The listing builds one solid part. Answer for the finished solid, in the listing's coordinates (mm). Face numbers are marked on the shaded views. Give positions to 0.01 mm unless a question says otherwise; leave off trailing zeros. Order: outer loops, then holes, each group sorted by start corner. A loop starts at its lowest first (then second) coordinate and runs counter-clockwise, first axis right, second up. Notation, with made-up numbers: (35.25, 56) - (65.25, 56) arc R28 cw to (65.25, 77) - close; hole circle Ø10 at (-20.5, 58.5). An arc over 180 degrees is marked (long way). Answer in a Markdown table with one row per item.
from build123d import *

# Parameters (mm, degrees)
BOSS_EXTRUDE2_DEPTH                                 = 5
CSK_FOR_M3_COUNTERSUNK_FLAT_HEAD_SCREW1_D           = 3.4
CSK_FOR_M3_COUNTERSUNK_FLAT_HEAD_SCREW1_DEPTH       = 5
CSK_FOR_M3_COUNTERSUNK_FLAT_HEAD_SCREW1_CSINK_D     = 6.3
CSK_FOR_M3_COUNTERSUNK_FLAT_HEAD_SCREW1_CSINK_ANGLE = 90
CSK_FOR_M3_COUNTERSUNK_FLAT_HEAD_SCREW1_TIP         = 1.021463052
CUT_EXTRUDE1_REACH                                  = 103.946
SKETCH4_W                                           = 16
SKETCH4_H                                           = 60
SKETCH5_R                                           = 25
CUT_EXTRUDE2_DEPTH                                  = 1
FILLET1_R                                           = 10


with BuildPart() as part:
    # Sketch1 → Boss-Extrude2 (new body)
    with BuildSketch(Plane.XY):
        with BuildLine():
            Line((-23.664319132, 68), (23.664319132, 68))
            ThreePointArc((23.664319132, 68), (0, -72), (-23.664319132, 68))
        make_face()
    extrude(amount=BOSS_EXTRUDE2_DEPTH)

    # Chamfer1: read off the stored shape, not the designer's step
    # Chamfer1 outline → Chamfer1 (revolve, cut)
    with BuildSketch(Plane.XZ):
        Polygon((72.000000172, 5.000000172), (67, 0), (72.000000172, 0), align=None)
    revolve(axis=Axis((0, 0, 0), (0, 0, 1)), mode=Mode.SUBTRACT)

    # CSK for M3 Countersunk Flat Head Screw1
    with Locations(Plane.XY.offset(5)):
        with Locations((15, -38.31), (-15, -38.31), (0, -52.31)):
            CounterSinkHole(CSK_FOR_M3_COUNTERSUNK_FLAT_HEAD_SCREW1_D / 2, CSK_FOR_M3_COUNTERSUNK_FLAT_HEAD_SCREW1_CSINK_D / 2, depth=CSK_FOR_M3_COUNTERSUNK_FLAT_HEAD_SCREW1_DEPTH, counter_sink_angle=CSK_FOR_M3_COUNTERSUNK_FLAT_HEAD_SCREW1_CSINK_ANGLE)
            with Locations((0, 0, -(CSK_FOR_M3_COUNTERSUNK_FLAT_HEAD_SCREW1_DEPTH + CSK_FOR_M3_COUNTERSUNK_FLAT_HEAD_SCREW1_TIP / 2))):  # 118° drill point
                Cone(0, CSK_FOR_M3_COUNTERSUNK_FLAT_HEAD_SCREW1_D / 2, CSK_FOR_M3_COUNTERSUNK_FLAT_HEAD_SCREW1_TIP, mode=Mode.SUBTRACT)

    # Cut-Extrude1: up to this face of the body (flat: up to its plane)
    cut_extrude1_end = Plane(part.part.faces().sort_by_distance((0, 0.083165236, 0))[0])
    # Sketch4 → Cut-Extrude1 (cut, up to the picked face)
    with BuildSketch(Plane.XY.offset(5), mode=Mode.PRIVATE) as cut_extrude1_sk1:
        with Locations((-0.5, 38)):
            Rectangle(SKETCH4_W, SKETCH4_H)
    cut_extrude1_tool1 = split(extrude(cut_extrude1_sk1.sketch, amount=-CUT_EXTRUDE1_REACH, mode=Mode.PRIVATE), bisect_by=cut_extrude1_end, keep=Keep.BOTH, mode=Mode.PRIVATE)
    add(cut_extrude1_tool1.solids().sort_by(Axis((-0.5, 38, 5), (0, 0, -1)))[0], mode=Mode.SUBTRACT)

    # Sketch5 → Cut-Extrude2 (cut)
    with BuildSketch(Plane.XY.offset(5)):
        with Locations((0, 61.9)):
            Circle(SKETCH5_R)
    extrude(amount=-CUT_EXTRUDE2_DEPTH, mode=Mode.SUBTRACT)

    # Fillet1
    # the kernel refuses this fillet: 10 mm, written as the material it adds along each edge
    with BuildSketch(Plane(origin=(-8.5, 8, 5), x_dir=(1, 0, 0), z_dir=(0, 0, -1)), Plane(origin=(7.5, 8, 5), x_dir=(0, 1, 0), z_dir=(0, 0, -1))) as fillet1_piece_1:
        with BuildLine():
            CenterArc((FILLET1_R, -FILLET1_R), FILLET1_R, 90, 90)
            Line((0, -FILLET1_R), (0, 0))
            Line((0, 0), (FILLET1_R, 0))
        make_face()
    extrude(amount=5)


solid = part.part
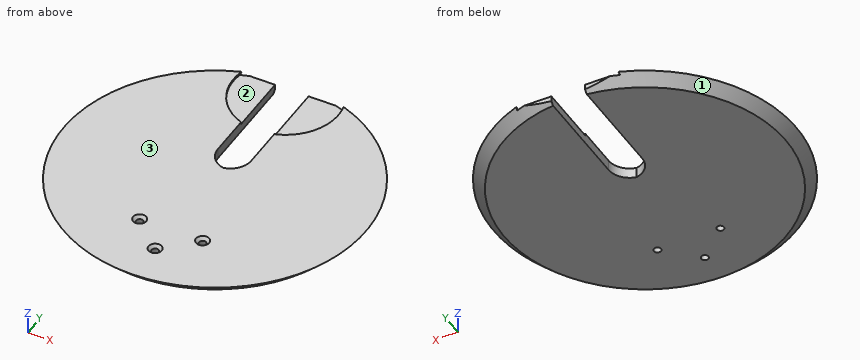
Item 1: Consider line 1 (X direction, y = -38.31, z = 0.8); line 2 (X direction, y = 47, z = 3.05); line 3 (X direction, y = -38.31, z = 2.35). Determine where each line is inside the solid, lowest interval first.
Answer block:
| item | result |
|---|---|
| line 1 | -55.94 to -16.7, -13.3 to 13.3, 16.7 to 55.94 |
| line 2 | -51.94 to -8.5, 7.5 to 51.94 |
| line 3 | -57.81 to -16.7, -13.3 to 13.3, 16.7 to 57.81 |
Item 2: Find section A-A on y = 0. Write down the section's boundary in (x, z).
Answer block:
| item | result |
|---|---|
| outline | (-72, 5) - (-67, 0) - (67, 0) - (72, 5) - close |
Item 3: Find section B-B on y = -38.31. Count the separate pieces of the cut face and the enclosed holes in it, then the cut area to 3 significant figures.
Answer block:
| item | result |
|---|---|
| separate pieces | 3 |
| enclosed holes | 0 |
| area | 542 mm² |
Item 4: Each of these flat-tipped pins is pushed along its axis until it touches: P1, Ø5.5, axis at x = 0, y = -52.31, coming from the +Z side; P2, Ø4.5, axis at x = 15, y = -38.31, coming from the +Z side; P3, Ø8, axis at x = -14, y = 49.5, coming from the +Z side; P4, Ø2, axis at x = -15, y = -38.31, coming from the -Z side. Where does it stop, or does it pass through?
Answer block:
| item | result |
|---|---|
| P1 | z = 4.6 |
| P2 | z = 4.1 |
| P3 | z = 4 |
| P4 | through |
Item 5: Determine the mould class of the marked faces 1, 2 and 3 for opening direction X: pulls with the +X half, pulls with the -X half, needs draft (parallel to the pull), parting line crosses it, or undercut.
Answer block:
| item | result |
|---|---|
| face 1 | parting line crosses it |
| face 2 | undercut |
| face 3 | needs draft |
